Part model, mm, in its own coordinate system. A direction names the side the tool comes from. Round coordinates to 2 decimals unless told otherwise and drop trailing zeros. Order: outer loops, then holes, each group sorted by start corner. A loop starts at its lowest first (then second) coordinate and runs counter-clockwise, first axis right, second up. Notation, with made-up numbers: (-30.75, 20) -> (-26.75, 20) arc R30 cw to (-26.75, 50) -> close; hole circle Ø5 at (88.25, 46.25). An arc over 180 degrees is marked (long way). Answer as a JSON object with one key per item and string values. Group by question number.
```python
from build123d import *

# Parameters (mm, degrees)
SKETCH1_R           = 11
SKETCH1_R_2         = 4.25
BOSS_EXTRUDE1_DEPTH = 4
SKETCH2_R           = 1.4
CUT_EXTRUDE1_DEPTH  = 17.062378404
SKETCH3_R           = 7.5
BOSS_EXTRUDE2_DEPTH = 2
SKETCH4_R           = 2.811136831
CUT_EXTRUDE2_DEPTH  = 2
SKETCH5_R           = 4.5
BOSS_EXTRUDE3_DEPTH = 7
CUT_EXTRUDE3_START  = -6
SKETCH6_R           = 4.5
SKETCH6_R_2         = 4
CUT_EXTRUDE3_DEPTH  = 6
BOSS_EXTRUDE4_DEPTH = 4
SKETCH13_W          = 22
SKETCH13_H          = 3.5
BOSS_EXTRUDE5_DEPTH = 46.25
SKETCH14_W          = 22
SKETCH14_H          = 5.5
BOSS_EXTRUDE6_DEPTH = 45
CUT_EXTRUDE6_START  = -30
SKETCH16_R          = 4.25
SKETCH16_R_2        = 1.4
CUT_EXTRUDE6_DEPTH  = 30
SKETCH17_W          = 10
SKETCH17_H          = 5.5
BOSS_EXTRUDE7_DEPTH = 20
SKETCH18_R          = 1.7
CUT_EXTRUDE7_DEPTH  = 30
FILLET2_R           = 3
FILLET3_R           = 2
SKETCH19_R          = 2.5
CUT_EXTRUDE8_DEPTH  = 1.5
CUT_EXTRUDE9_DEPTH  = 3


with BuildPart() as part:
    # Sketch1 → Boss-Extrude1 (new body)
    with BuildSketch(Plane(origin=(0, 0, 0), x_dir=(1, 0, 0), z_dir=(0, 1, 0))):
        with Locations(Location((0, 0, 0), (0, 0, 270))):
            Circle(SKETCH1_R)
        with Locations(Location((0, 0, 0), (0, 0, 270))):
            Circle(SKETCH1_R_2, mode=Mode.SUBTRACT)
    extrude(amount=BOSS_EXTRUDE1_DEPTH)

    # Sketch2 → Cut-Extrude1 (cut, through all)
    with BuildSketch(Plane(origin=(0, 4, 0), x_dir=(1, 0, 0), z_dir=(0, 1, 0))):
        with Locations(Location((0, 8, 0), (0, 0, 270))):
            Circle(SKETCH2_R)
        with Locations(Location((8, 0, 0), (0, 0, 270))):
            Circle(SKETCH2_R)
        with Locations(Location((0, -8, 0), (0, 0, 270))):
            Circle(SKETCH2_R)
        with Locations(Location((-8, 0, 0), (0, 0, 270))):
            Circle(SKETCH2_R)
    extrude(amount=-CUT_EXTRUDE1_DEPTH, mode=Mode.SUBTRACT)

    # Sketch3 → Boss-Extrude2 (add)
    with BuildSketch(Plane(origin=(0, 4, 0), x_dir=(1, 0, 0), z_dir=(0, 1, 0))):
        with Locations(Location((0, 0, 0), (0, 0, 80.315835906))):
            Circle(SKETCH3_R)
    extrude(amount=BOSS_EXTRUDE2_DEPTH)

    # Sketch4 → Cut-Extrude2 (cut)
    with BuildSketch(Plane(origin=(0, 6, 0), x_dir=(1, 0, 0), z_dir=(0, 1, 0))):
        with Locations((8, 0)):
            Circle(SKETCH4_R)
        with Locations((0, -8)):
            Circle(SKETCH4_R)
        with Locations((-8, 0)):
            Circle(SKETCH4_R)
        with Locations((0, 8)):
            Circle(SKETCH4_R)
    extrude(amount=-CUT_EXTRUDE2_DEPTH, mode=Mode.SUBTRACT)

    # Sketch5 → Boss-Extrude3 (add)
    with BuildSketch(Plane(origin=(0, 6, 0), x_dir=(1, 0, 0), z_dir=(0, 1, 0))):
        with Locations(Location((0, 0, 0), (0, 0, 270))):
            Circle(SKETCH5_R)
    extrude(amount=BOSS_EXTRUDE3_DEPTH)

    # Sketch6 → Cut-Extrude3 (cut)
    with BuildSketch(Plane(origin=(0, 13, 0), x_dir=(1, 0, 0), z_dir=(0, 1, 0)).offset(CUT_EXTRUDE3_START)):
        with Locations(Location((0, 0, 0), (0, 0, 270))):
            Circle(SKETCH6_R)
        with Locations(Location((0, 0, 0), (0, 0, 270))):
            Circle(SKETCH6_R_2, mode=Mode.SUBTRACT)
    extrude(amount=CUT_EXTRUDE3_DEPTH, mode=Mode.SUBTRACT)

    # Sketch8 → Boss-Extrude4 (add)
    with BuildSketch(Plane.XZ):
        with BuildLine():
            Line((11, 30), (-11, 30))
            Line((-11, 30), (-11, 0))
            ThreePointArc((-11, 0), (0, 11), (11, 0))
            Line((11, 0), (11, 30))
        make_face()
    extrude(amount=-BOSS_EXTRUDE4_DEPTH)

    # Sketch13 → Boss-Extrude5 (add)
    with BuildSketch(Plane(origin=(0, 4, 0), x_dir=(1, 0, 0), z_dir=(0, 1, 0))):
        with Locations((0, -31.75)):
            Rectangle(SKETCH13_W, SKETCH13_H)
    extrude(amount=-BOSS_EXTRUDE5_DEPTH)

    # Sketch14 → Boss-Extrude6 (add)
    with BuildSketch(Plane.XY.offset(33.5)):
        with Locations((0, -45)):
            Rectangle(SKETCH14_W, SKETCH14_H)
    extrude(amount=-BOSS_EXTRUDE6_DEPTH)

    # Sketch16 → Cut-Extrude6 (cut)
    with BuildSketch(Plane.XZ.offset(47.75).offset(CUT_EXTRUDE6_START)):
        with Locations(Location((0, 0, 0), (0, 0, 90))):
            Circle(SKETCH16_R)
        with Locations(Location((-8, 0, 0), (0, 0, 90))):
            Circle(SKETCH16_R_2)
        with Locations(Location((0, -8, 0), (0, 0, 90))):
            Circle(SKETCH16_R_2)
        with Locations(Location((8, 0, 0), (0, 0, 90))):
            Circle(SKETCH16_R_2)
        with Locations(Location((0, 8, 0), (0, 0, 90))):
            Circle(SKETCH16_R_2)
    extrude(amount=CUT_EXTRUDE6_DEPTH, mode=Mode.SUBTRACT)

    # Sketch17 → Boss-Extrude7 (add)
    with BuildSketch(Plane(origin=(0, 0, -11.5), x_dir=(-1, 0, 0), z_dir=(0, 0, -1))):
        with Locations((-16, -45)):
            Rectangle(SKETCH17_W, SKETCH17_H)
        with Locations((16, -45)):
            Rectangle(SKETCH17_W, SKETCH17_H)
    extrude(amount=-BOSS_EXTRUDE7_DEPTH)

    # Sketch18 → Cut-Extrude7 (cut)
    with BuildSketch(Plane(origin=(0, -47.75, 0), x_dir=(-1, 0, 0), z_dir=(0, -1, 0))):
        with Locations(Location((16, -3.5, 0), (0, 0, 90))):
            Circle(SKETCH18_R)
        with Locations(Location((16, 6.5, 0), (0, 0, 90))):
            Circle(SKETCH18_R)
        with Locations(Location((-16, 6.5, 0), (0, 0, 270))):
            Circle(SKETCH18_R)
        with Locations(Location((-16, -3.5, 0), (0, 0, 270))):
            Circle(SKETCH18_R)
    extrude(amount=-CUT_EXTRUDE7_DEPTH, mode=Mode.SUBTRACT)

    # Fillet2
    fillet2_edges = [part.edges().sort_by_distance(p)[0] for p in [
        (21, -45, 8.5),
        (11, -45, 8.5),
        (21, -45, -11.5),
        (-21, -45, 8.5),
        (-11, -45, 8.5),
        (-21, -45, -11.5),
    ]]
    fillet(fillet2_edges, radius=FILLET2_R)

    # Fillet3
    fillet3_edges = [part.edges().sort_by_distance(p)[0] for p in [
        (0, 0, 30),
        (0, -42.25, 30),
        (0, 4, 33.5),
        (0, -47.75, 33.5),
    ]]
    fillet(fillet3_edges, radius=FILLET3_R)

    # Sketch19 → Cut-Extrude8 (cut)
    with BuildSketch(Plane.XZ.offset(47.75)):
        with Locations((-8, 0)):
            Circle(SKETCH19_R)
        with Locations((0, 8)):
            Circle(SKETCH19_R)
        with Locations((8, 0)):
            Circle(SKETCH19_R)
        with Locations((0, -8)):
            Circle(SKETCH19_R)
    extrude(amount=-CUT_EXTRUDE8_DEPTH, mode=Mode.SUBTRACT)

    # Sketch20 → Cut-Extrude9 (cut)
    with BuildSketch(Plane(origin=(0, -42.25, 0), x_dir=(1, 0, 0), z_dir=(0, 1, 0))):
        Polygon((17.674315781, 3.6), (19.348631561, 6.5), (17.674315781, 9.4), (14.325684219, 9.4), (12.651368439, 6.5), (14.325684219, 3.6), align=None)
        Polygon((-14.325684219, 3.6), (-12.651368439, 6.5), (-14.325684219, 9.4), (-17.674315781, 9.4), (-19.348631561, 6.5), (-17.674315781, 3.6), align=None)
        Polygon((17.674315781, -6.4), (19.348631561, -3.5), (17.674315781, -0.6), (14.325684219, -0.6), (12.651368439, -3.5), (14.325684219, -6.4), align=None)
        Polygon((-14.325684219, -6.4), (-12.651368439, -3.5), (-14.325684219, -0.6), (-17.674315781, -0.6), (-19.348631561, -3.5), (-17.674315781, -6.4), align=None)
    extrude(amount=-CUT_EXTRUDE9_DEPTH, mode=Mode.SUBTRACT)


solid = part.part
```
Q1. Which spindle directions (+Z, -Z, +X, -X, +Y, -Y) get a long thin tool onto all of the face, cutting with end or side? Do faces 1 (the flat face through (-13.5, -43.73, 4.97)), 2 (the cylindrical face through (-0.54, -47.01, -10.44)), 3 (the cylindrical face through (-0.05, 5.01, -5.19)). Say none if no direction does.
Q2. Band-saw the part on D-D (x = -8). List the corners of the cut face in (y, z).
Q3. Band-saw the part on B-B (x = -16). List the corners of the cut face in (y, z), plus the area to 3 significant figures.
Q4. Two-plate mould, pull along X, no slides. Class faces 4 (the cylindrical face through (20.14, -44.96, 7.6)), 5 (the flat face through (-16, -44, -3.6)), 6 (the flat face through (-11, -20.1, 30.5)): +X half, -X half, draft (parallel to the pull), parting line (faces both ways), or undercut.
Q5. Wall check: line 1 (Y direction, x = 1.5, z = -8); line 2 (Y direction, x = 1, z = 25); line 3 (Z direction, x = 19, y = -43.5). Give the ranges that are in metal, low to high. Write a range as [from, to].
Q6. Band-saw the part on C-C (y = -28.5). List the corners of the cut face in (x, z).
Q7. Drop flat-ended pins along their axis: pin 1 Ø1 at (x, z) = (-5.5, 10) entering from +Y; pin 2 Ø11 at (x, y) = (5, -20.5) entering from -Z; pin 3 Ø3 at (x, y) = (-15.5, -44) entering from +Z. Give the stop position or say it passes through.
Q8. Band-saw the part on A-A (z = 22.5). List the corners of the cut face in (x, y).
Completed:
{
 "1": {"face 1": "+Y", "face 2": "-Y", "face 3": "-Z, +Y"},
 "2": {"outline": "(-47.75, -11.5) -> (-42.25, -11.5) -> (-42.25, -1.4) -> (-46.25, -1.4) -> (-46.25, -2.5) -> (-47.75, -2.5) -> close; (-47.75, 2.5) -> (-46.25, 2.5) -> (-46.25, 1.4) -> (-42.25, 1.4) -> (-42.25, 28) arc R2 cw to (-40.25, 30) -> (-2, 30) arc R2 cw to (0, 28) -> (0, 1.4) -> (4, 1.4) -> (4, 31.5) arc R2 ccw to (2, 33.5) -> (-45.75, 33.5) arc R2 ccw to (-47.75, 31.5) -> close; (0, -7.55) -> (4, -7.55) -> (4, -1.4) -> (0, -1.4) -> close"},
 "3": {"outline": "(-47.75, -11.5) -> (-42.25, -11.5) -> (-42.25, -9.4) -> (-45.25, -9.4) -> (-45.25, -8.2) -> (-47.75, -8.2) -> close; (-47.75, -4.8) -> (-45.25, -4.8) -> (-45.25, -3.6) -> (-42.25, -3.6) -> (-42.25, 0.6) -> (-45.25, 0.6) -> (-45.25, 1.8) -> (-47.75, 1.8) -> close; (-47.75, 5.2) -> (-45.25, 5.2) -> (-45.25, 6.4) -> (-42.25, 6.4) -> (-42.25, 8.5) -> (-47.75, 8.5) -> close", "area": "58.2 mm2"},
 "4": {"face 4": "+X half", "face 5": "undercut", "face 6": "-X half"},
 "5": {"line 1": "[-46.25, -42.25], [0, 4]", "line 2": "[-47.75, -42.25], [0, 4]", "line 3": "[-11.33, -7.1], [-5.9, 2.9], [4.1, 8.33]"},
 "6": {"outline": "(-11, 30) -> (11, 30) -> (11, 33.5) -> (-11, 33.5) -> close"},
 "7": {"pin 1": "y = 4", "pin 2": "z = 30", "pin 3": "z = 8.5"},
 "8": {"outline": "(-11, -47.75) -> (11, -47.75) -> (11, -42.25) -> (-11, -42.25) -> close; (-11, 0) -> (11, 0) -> (11, 4) -> (-11, 4) -> close"}
}
